Read the model definition and answer for the solid it produces. Units are mm, in the model's axes. Face numbers are marked on the shaded views. A direction names the side the tool comes from. Give positions to 0.01 mm unless a question says otherwise; leave off trailing zeros. Order: outer loops, then holes, each group sorted by start corner. A loop starts at its lowest first (then second) coordinate and runs counter-clockwise, first axis right, second up. Notation, with made-up numbers: M -11,71.5 L 42,71.5 A26 cw 42,89.5 Z; hole C 27,-28.75 d2. An arc over 180 degrees is marked long. Write item = value, one per line. Start each with the question number.
from build123d import *

# Parameters (mm, degrees)
SKETCH1_R               = 25.4
SKETCH1_R_2             = 5.08
BOSS_EXTRUDE1_DEPTH     = 19.05
BOSS_EXTRUDE2_START     = 6.35
SKETCH4_R               = 12.7
SKETCH4_R_2             = 5.08
BOSS_EXTRUDE2_DEPTH     = 6.35
CUT_EXTRUDE1_REACH      = 51.595
CUT_EXTRUDE1_END_RADIUS = 5.08
SKETCH5_R               = 1.27


with BuildPart() as part:
    # Sketch1 → Boss-Extrude1 (new body)
    with BuildSketch(Plane.XY):
        with Locations(Location((0, 0, 0), (0, 0, 180))):
            Circle(SKETCH1_R)
        with Locations(Location((0, 0, 0), (0, 0, 180))):
            Circle(SKETCH1_R_2, mode=Mode.SUBTRACT)
    extrude(amount=BOSS_EXTRUDE1_DEPTH)

    # Sketch3 → Cut-Revolve1 (revolve, cut)
    with BuildSketch(Plane(origin=(0, 0, 0), x_dir=(0, 0, -1), z_dir=(1, 0, 0)), mode=Mode.PRIVATE) as cut_revolve1_sk:
        Polygon((0, 25.4), (0, 34.911662418), (-19.05, 34.911662418), (-19.05, 25.4), (-13.335, 17.78), (-5.715, 17.78), align=None)
    revolve(cut_revolve1_sk.sketch.rotate(Axis((0, 0, 21.061205324), (0, 0, -1)), 90), axis=Axis((0, 0, 21.061205324), (0, 0, -1)), mode=Mode.SUBTRACT)

    # Sketch4 → Boss-Extrude2 (add)
    with BuildSketch(Plane(origin=(0, 0, 0), x_dir=(-1, 0, 0), z_dir=(0, 0, -1)).offset(BOSS_EXTRUDE2_START)):
        with Locations(Location((0, 0, 0), (0, 0, 180))):
            Circle(SKETCH4_R)
        Circle(SKETCH4_R_2, mode=Mode.SUBTRACT)
    extrude(amount=-BOSS_EXTRUDE2_DEPTH)

    # Cut-Extrude1: up to this cylinder (the profile starts outside it)
    cut_extrude1_end = Plane(origin=(0, 0, -3.175), z_dir=(0, 0, -1)) * Cylinder(CUT_EXTRUDE1_END_RADIUS, 114.35, mode=Mode.PRIVATE)
    # Sketch5 → Cut-Extrude1 (cut, up to the surface)
    with BuildSketch(Plane(origin=(12.7, 0, 0), x_dir=(0, 0, -1), z_dir=(1, 0, 0)), mode=Mode.PRIVATE) as cut_extrude1_sk1:
        with Locations((3.175, 0)):
            Circle(SKETCH5_R)
    cut_extrude1_tool1 = extrude(cut_extrude1_sk1.sketch, amount=-CUT_EXTRUDE1_REACH, mode=Mode.PRIVATE) - cut_extrude1_end
    add(cut_extrude1_tool1.solids().sort_by_distance((12.7, 0, -3.175))[0], mode=Mode.SUBTRACT)


solid = part.part
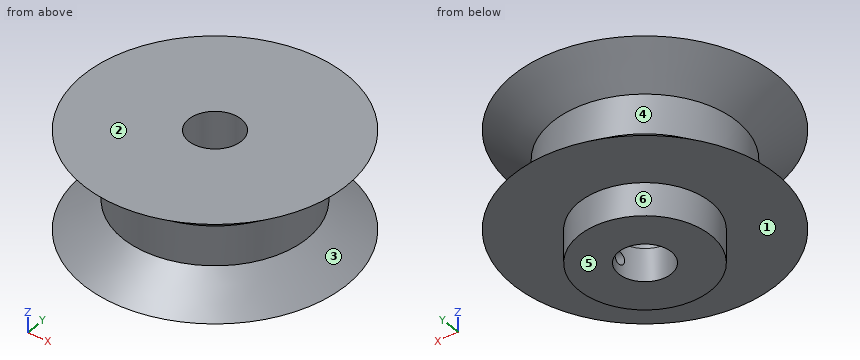
1) For the marked faces 4, 5 and 6, determine the directions among +Z, -Z, +X, -X, +Y, -Y from which every point of the face is accessible in a straight line to the end or side of a thin tool.
2) Find the intervals of material crossed by probe 1 along Y at (x, z) = (0, -2.5); probe 2 along Y at (x, z) = (0, 9.25), in increasing order. Write a range as [from, to].
3) For a pull along Z with two mould halves and no side action, classify the marked faces 1, 2 and 3 as pulls with the +Z half, pulls with the -Z half, needs draft (parallel to the pull), parting line crosses it, or undercut.
4) Each of these flat-tipped pins is pushed along its axis until it touches: P1, Ø2, axis at y = 13, z = 5, coming from the -X side; P2, Ø1, axis at y = 0.5, z = 6.5, coming from the -X side; P3, Ø6, axis at x = -14.5, y = 18.5, coming from the -Z side. Where does it stop, or does it pass through?
5) Find section A-A on x = 0. Determine the outline of the cut face in (y, z) (3 decimals).
6) Find section B-B on y = 0. Determine the outline of the cut face in (x, z) (3 decimals), plus the area to 3 significant figures.
Numbers:
q1.face_4 = none
q1.face_5 = -Z, +X, -X, +Y, -Y
q1.face_6 = -Z
q2.probe_1 = [-12.7, -5.08], [5.08, 12.7]
q2.probe_2 = [-17.78, -5.08], [5.08, 17.78]
q3.face_1 = pulls with the -Z half
q3.face_2 = pulls with the +Z half
q3.face_3 = undercut
q4.P1 = -15.48
q4.P2 = -17.78
q4.P3 = 0
q5.outline = M -25.4,0 L -12.7,0 L -12.7,-6.35 L -5.08,-6.35 L -5.08,19.05 L -25.4,19.05 L -17.78,13.335 L -17.78,5.715 Z; M 5.08,-6.35 L 12.7,-6.35 L 12.7,0 L 25.4,0 L 17.78,5.715 L 17.78,13.335 L 25.4,19.05 L 5.08,19.05 Z
q6.outline = M -25.4,0 L -12.7,0 L -12.7,-6.35 L -5.08,-6.35 L -5.08,19.05 L -25.4,19.05 L -17.78,13.335 L -17.78,5.715 Z; M 5.08,-6.35 L 12.7,-6.35 L 12.7,-4.445 L 5.08,-4.445 Z; M 5.08,-1.905 L 12.7,-1.905 L 12.7,0 L 25.4,0 L 17.78,5.715 L 17.78,13.335 L 25.4,19.05 L 5.08,19.05 Z
q6.area = 648 mm2
